Check sheet for the modelled part. Datum: model origin and axes. Units: mm. Face numbers are marked on the shaded views. A direction names the side the tool comes from. Give positions to 0.01 mm unless a question says otherwise; leave off trailing zeros. Write each loop counter-clockwise with the first axis right and the second up, starting at its lowest first coordinate (ties: lowest second). Pieces come first, ordered by that corner, then holes.
from build123d import *

# Parameters (mm, degrees)
SKETCH1_W           = 140
SKETCH1_H           = 100.00000000000001
BOSS_EXTRUDE1_DEPTH = 55
CUT_EXTRUDE1_DEPTH  = 17
SKETCH3_W           = 5.800000000000001
SKETCH3_H           = 5.340000000000003
SKETCH3_W_2         = 5.799999999999969
CUT_EXTRUDE2_DEPTH  = 13.4
CUT_EXTRUDE3_DEPTH  = 17
SHELL1_T            = -4
CUT_EXTRUDE4_DEPTH  = 177.19307591389622
CUT_EXTRUDE5_DEPTH  = 181.62391868188442
SKETCH9_W           = 48.000000000000014
SKETCH9_H           = 14.000000000000002
CUT_EXTRUDE6_DEPTH  = 181.62391868188442
CUT_EXTRUDE7_DEPTH  = 4


with BuildPart() as part:
    # Sketch1 → Boss-Extrude1 (new body)
    with BuildSketch(Plane(origin=(0, 0, 0), x_dir=(1, 0, 0), z_dir=(0, 1, 0))):
        with Locations((70, 50.00000000000001)):
            Rectangle(SKETCH1_W, SKETCH1_H)
    extrude(amount=BOSS_EXTRUDE1_DEPTH)

    # Sketch2 → Cut-Extrude1 (cut)
    with BuildSketch(Plane(origin=(0, 55, 0), x_dir=(1, 0, 0), z_dir=(0, 1, 0))):
        Polygon((6.000000000000011, 85), (28.50000000000001, 84.99999999999999), (28.50000000000001, 15.000000000000014), (6.000000000000011, 15), align=None)
        Polygon((134.00000000000003, 15.000000000000014), (111.50000000000003, 15.000000000000023), (111.5, 85), (134, 85.00000000000001), align=None)
    extrude(amount=-CUT_EXTRUDE1_DEPTH, mode=Mode.SUBTRACT)

    # Sketch3 → Cut-Extrude2 (cut)
    with BuildSketch(Plane(origin=(0, 55, 0), x_dir=(1, 0, 0), z_dir=(0, 1, 0))):
        with Locations((17.250000000000014, 87.66999999999999)):
            Rectangle(SKETCH3_W, SKETCH3_H)
        with Locations((122.74999999999997, 87.67)):
            Rectangle(SKETCH3_W_2, SKETCH3_H)
    extrude(amount=-CUT_EXTRUDE2_DEPTH, mode=Mode.SUBTRACT)

    # Sketch4 → Cut-Extrude3 (cut)
    with BuildSketch(Plane(origin=(0, 55, 0), x_dir=(1, 0, 0), z_dir=(0, 1, 0))):
        Polygon((3.2500000000000098, 31.5), (31.250000000000014, 31.5), (31.250000000000014, 11.5), (3.2500000000000115, 11.5), align=None)
        Polygon((136.75, 11.500000000000016), (108.75000000000003, 11.500000000000009), (108.75000000000001, 31.500000000000007), (136.75000000000003, 31.500000000000014), align=None)
    extrude(amount=-CUT_EXTRUDE3_DEPTH, mode=Mode.SUBTRACT)

    # Shell1
    shell1_openings = [part.faces().sort_by_distance(p)[0] for p in [
        (70, 0, -50),
    ]]
    offset(amount=SHELL1_T, openings=shell1_openings, kind=Kind.INTERSECTION)

    # Sketch5 → Cut-Extrude4 (cut, through all)
    with BuildSketch(Plane(origin=(0, 38, 0), x_dir=(1, 0, 0), z_dir=(0, 1, 0))):
        Polygon((7.25000000000001, 36.5), (27.250000000000014, 36.5), (27.25000000000001, 18.5), (7.2500000000000115, 18.5), align=None)
        Polygon((132.75000000000003, 18.500000000000014), (112.75000000000001, 18.50000000000001), (112.75000000000001, 36.500000000000014), (132.75000000000003, 36.500000000000014), align=None)
    extrude(amount=-CUT_EXTRUDE4_DEPTH, mode=Mode.SUBTRACT)

    # Sketch6 → Cut-Extrude5 (cut, through all)
    with BuildSketch(Plane(origin=(0, 55, 0), x_dir=(1, 0, 0), z_dir=(0, 1, 0))):
        Polygon((57.24999999999999, 31.38695956479682), (82.75000000000001, 31.38695956479682), (82.75, 18.98695956479682), (57.25000000000001, 18.98695956479682), align=None)
    extrude(amount=-CUT_EXTRUDE5_DEPTH, mode=Mode.SUBTRACT)

    # Sketch9 → Cut-Extrude6 (cut, through all)
    with BuildSketch(Plane(origin=(140, 0, 0), x_dir=(0, 0, -1), z_dir=(1, 0, 0))):
        with Locations((50.00000000000001, 7.000000000000001)):
            Rectangle(SKETCH9_W, SKETCH9_H)
    extrude(amount=-CUT_EXTRUDE6_DEPTH, mode=Mode.SUBTRACT)

    # Sketch8 → Cut-Extrude7 (cut)
    with BuildSketch(Plane.XY):
        Polygon((64, 5.2e-15), (76.00000000000001, 5.2e-15), (76.00000000000001, 8.000000000000004), (64, 8), align=None)
    extrude(amount=-CUT_EXTRUDE7_DEPTH, mode=Mode.SUBTRACT)


solid = part.part
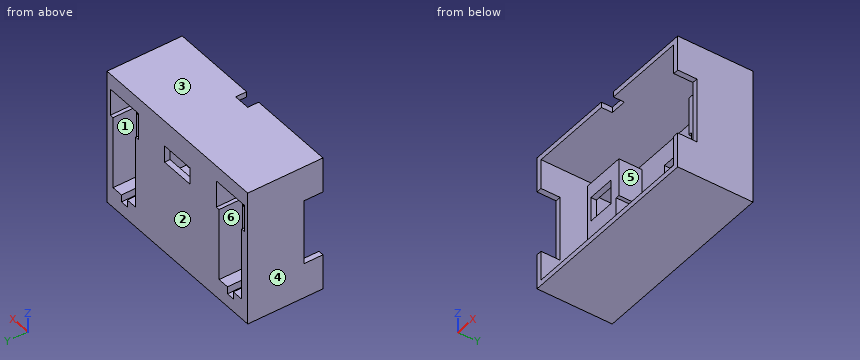
1) Sectioned sample at D-D on y = 32. Record the boundary of the cut face in (x, z), then the cut area to 3 significant figures.
2) Sectioned sample at A-A on x = 61. Record the boundary of the cut face in (y, z), then the cut area to 3 significant figures.
3) Draft check along Z on the marked faces 1, 2 and 3. Enter one of: +Z half, -Z half, draft (parallel to the pull), parting line (faces both ways), or undercut.
4) Access from +Z, -Z, +X, -X, +Y, -Y to the whole of each face (thin tool, end or side, straight path). Record for the marked faces 4, 5 and 6.
5) Sectioned sample at B-B on y = 10.5. Record the boundary of the cut face in (x, z).
6) Gauge pin test, flat ends, axial feed: pin 1 (12 mm diameter, centred on x = 66, z = -60.5, fed in from -Y); pin 2 (1.2 mm diameter, centred on x = 2, z = -38.5, fed in from -Y); pin 3 (1.2 mm diameter, centred on x = 67.5, z = -3, fed in from -Y). Record the tip position at first contact, or that the pin passes through.
7) Sectioned sample at C-C on z = -62.5. Record the boundary of the cut face in (x, y), then the cut area to 3 significant figures.
8) Scan lines: L1, parallel to Z at x = 116.5, y = 41.5; L2, parallel to Z at x = 17, y = 37; L3, parallel to X at y = 47, z = -47. Record each from-to range of solid material in increasing order.
Answers below:
1. outline: (0, -100) - (140, -100) - (140, 0) - (0, 0) - close; hole (4, -96) - (136, -96) - (136, -4) - (4, -4) - close
1. area: 1,860 mm2
2. outline: (0, -100) - (55, -100) - (55, -31.39) - (51, -31.39) - (51, -96) - (0, -96) - close; (0, -4) - (51, -4) - (51, -18.99) - (55, -18.99) - (55, 0) - (0, 0) - close
2. area: 758 mm2
3. face 1: undercut
3. face 2: draft
3. face 3: +Z half
4. face 4: +Z, -Z, -X, +Y, -Y
4. face 5: -Y
4. face 6: +Y
5. outline: (0, -100) - (140, -100) - (140, -74) - (136, -74) - (136, -96) - (4, -96) - (4, -74) - (0, -74) - close; (0, -26) - (4, -26) - (4, -4) - (136, -4) - (136, -26) - (140, -26) - (140, 0) - (0, 0) - close
6. pin 1: stops at y = 51
6. pin 2: stops at y = 14
6. pin 3: stops at y = 8
7. outline: (0, 14) - (4, 14) - (4, 34) - (32.5, 34) - (32.5, 51) - (107.5, 51) - (107.5, 34) - (136, 34) - (136, 14) - (140, 14) - (140, 55) - (134, 55) - (134, 38) - (111.5, 38) - (111.5, 55) - (28.5, 55) - (28.5, 38) - (6, 38) - (6, 55) - (0, 55) - close
7. area: 1,060 mm2
8. L1: z = -100 to -96, -94.34 to -85, -11.5 to -7.5, -4 to 0
8. L2: z = -100 to -96, -89 to -36.5, -18.5 to -7.5, -4 to 0
8. L3: x = 0 to 6, 28.5 to 32.5, 107.5 to 111.5, 134 to 140
